from build123d import *

# Parameters (mm, degrees)
SKETCH1_R           = 17.5
BOSS_EXTRUDE1_DEPTH = 37
SKETCH3_W           = 21.176447949
SKETCH3_H           = 25
CUT_EXTRUDE1_DEPTH  = 74
SKETCH4_R           = 5
CUT_EXTRUDE2_DEPTH  = 74
CUT_EXTRUDE3_DEPTH  = 74


with BuildPart() as part:
    # Sketch1 → Boss-Extrude1 (new, symmetric)
    with BuildSketch(Plane.XY):
        Circle(SKETCH1_R)
    extrude(amount=BOSS_EXTRUDE1_DEPTH, both=True)

    # Sketch3 → Cut-Extrude1 (cut)
    with BuildSketch(Plane.XY.offset(37)):
        with Locations((-22.835672689, 0)):
            Rectangle(SKETCH3_W, SKETCH3_H)
        with Locations((22.835672689, 0)):
            Rectangle(SKETCH3_W, SKETCH3_H)
    extrude(amount=-CUT_EXTRUDE1_DEPTH, mode=Mode.SUBTRACT)

    # Sketch4 → Cut-Extrude2 (cut)
    with BuildSketch(Plane.XY.offset(37)):
        Circle(SKETCH4_R)
    extrude(amount=-CUT_EXTRUDE2_DEPTH, mode=Mode.SUBTRACT)

    # Sketch5 → Cut-Extrude3 (cut)
    with BuildSketch(Plane(origin=(12.247448714, 0, 0), x_dir=(0, 0, -1), z_dir=(1, 0, 0))):
        Polygon((14.43375673, 0), (7.216878365, 12.5), (-7.216878365, 12.5), (-14.43375673, 0), (-7.216878365, -12.5), (7.216878365, -12.5), align=None)
    extrude(amount=-CUT_EXTRUDE3_DEPTH, mode=Mode.SUBTRACT)


solid = part.part
Here's how the part is built. I have some questions about the finished solid (model axes, mm). A direction names the side the tool comes from. Round coordinates to 2 decimals unless told otherwise and drop trailing zeros. Loops run counter-clockwise (first coordinate to the right, second up) from the corner with the lowest first, then second, coordinate; pieces in that order, holes last. Notation, with made-up numbers: M 26.25,16 L 45.25,16 A23 ccw 45.25,34 Z; hole C 77,17.25 d2. An arc over 180 degrees is marked long. Write each question's results on one line, items separated by ' | '. Start each with the question number.
(1) On a 3-axis mill with a long thin cutter (end or side, diameter ignored), from which of +Z, -Z, +X, -X, +Y, -Y can I reach the whole of each face in a straight line? I mean faces 1 (the flat face through (0.171, 6.162, -10.876)), 2 (the flat face through (-12.247, 0, 26)). Say none if no direction works.
(2) I want a section at D-D (x = -9.5). Please give me the cut outline in (y, z).
(3) Thinking about a two-plate mould opening in Z: for faces 3 (the flat face through (-6, 0, -37)), 4 (the flat face through (12.247, 0, 26)), 5 (the flat face through (0, -12.5, 0)), which applies, pulls with the +Z half, pulls with the -Z half, needs draft (parallel to the pull), parting line crosses it, or undercut?
(4) I want a section at C-C (z = -16.5). Please give me the cut outline in (x, y).
(5) Will these pins go through, and if not, where does the flat tip stop? P1, Ø5, axis at x = 3.5, z = 4.5, coming from the -Y side; P2, Ø2, axis at x = -4.5, z = -26, coming from the -Y side; P3, Ø3, axis at x = 3.5, z = -14.5, coming from the +Y side.
(6) If I drill on probe 1 along X at (y, z) = (0, -19); probe 2 along Y at (x, z) = (0.25, -32.5); probe 3 along Z at (x, y) = (-10.5, -5), over which ranges is the centre line in solid material (lowest first)? Write a range as from..to.
(7) I want a section at A-A (x = 0). Please give me the cut outline in (y, z).
(8) I want a section at B-B (y = 9.5). Please give me the cut outline in (x, z).
Solved:
1) face 1: +X, -X | face 2: +Z, -Z, -X, +Y, -Y
2) outline: M -14.7,-37 L 14.7,-37 L 14.7,37 L -14.7,37 Z; hole M -12.5,-7.22 L 0,-14.43 L 12.5,-7.22 L 12.5,7.22 L 0,14.43 L -12.5,7.22 Z
3) face 3: pulls with the -Z half | face 4: needs draft | face 5: undercut
4) outline: M -12.25,-12.5 A17.5 ccw 12.25,-12.5 L 12.25,12.5 A17.5 ccw -12.25,12.5 Z; hole C 0,0 d10
5) P1: stops at y = -17.47 | P2: stops at y = -17.15 | P3: stops at y = 17.39
6) probe 1: x = -12.25..-5, 5..12.25 | probe 2: y = -17.5..-4.99, 4.99..17.5 | probe 3: z = -37..-11.55, 11.55..37
7) outline: M -17.5,-37 L -5,-37 L -5,-11.55 L -12.5,-7.22 L -12.5,7.22 L -5,11.55 L -5,37 L -17.5,37 Z; M 5,-37 L 17.5,-37 L 17.5,37 L 5,37 L 5,11.55 L 12.5,7.22 L 12.5,-7.22 L 5,-11.55 Z
8) outline: M -12.25,-37 L 12.25,-37 L 12.25,-8.95 L -12.25,-8.95 Z; M -12.25,8.95 L 12.25,8.95 L 12.25,37 L -12.25,37 Z
